The drawing under review shows one solid part. Ordinate dimensions are in mm from its lowest x, y, z. Give positions to 0.01 mm unless a question says otherwise; leave off trailing zeros. Write each loop counter-clockwise with the first axis right and the second up, starting at its lowest first coordinate (ties: lowest second). Pieces come first, ordered by that corner, then holes. Notation, with made-up numbers: (12.5, 4) -> (45.5, 4) arc R36 cw to (45.5, 38) -> close; hole circle Ø2 at (-16, -3.75). An arc over 180 degrees is marked (long way). Answer as a JSON object with one key per item and string values.
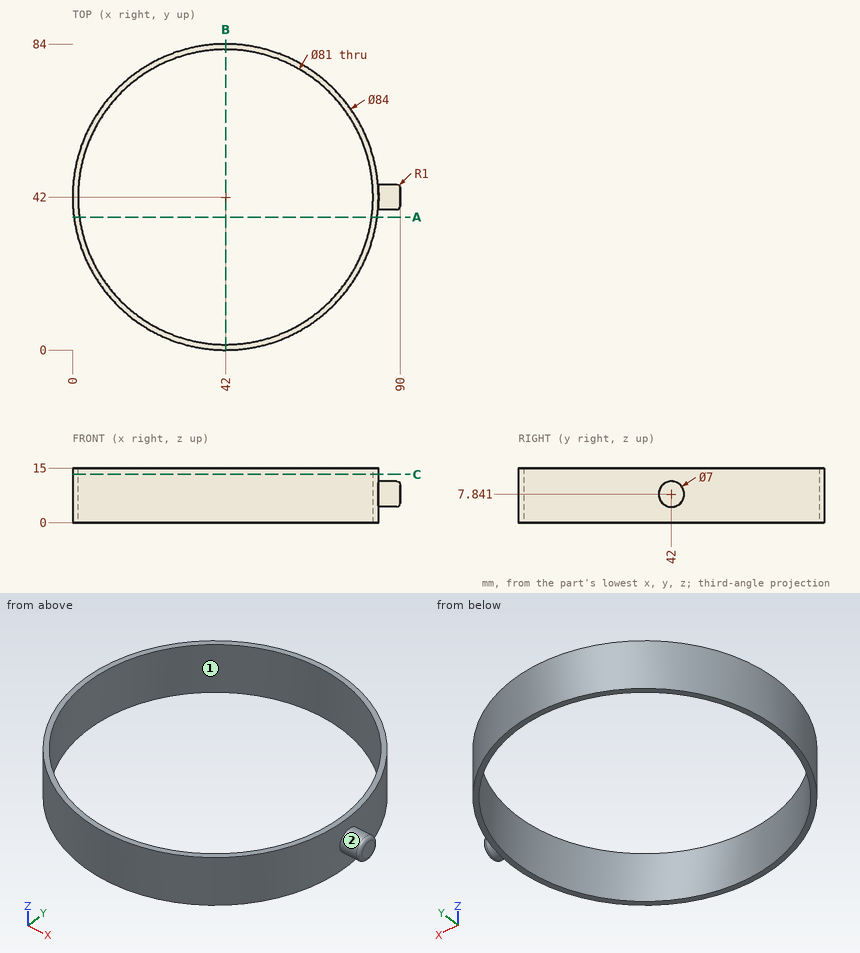
(1) We need section B-B, the plane x = 42. State the section outline as (y, z) points, then the cut area to 3 significant figures.
Here are the results:
{"outline": "(0, 0) -> (1.5, 0) -> (1.5, 15) -> (0, 15) -> close; (82.5, 0) -> (84, 0) -> (84, 15) -> (82.5, 15) -> close", "area": "45.0 mm²"}
(2) For line 1 along Y through (x, z) = (42, 7); line 2 along Y through (x, z) = (54, 7.75); line 3 along X through (y, z) = (52, 10.5) (1 decimal), list the stretches that pass through material, from the lowest coordinate up.
Here are the results:
{"line 1": "y = 0 to 1.5, 82.5 to 84", "line 2": "y = 1.75 to 3.32, 80.68 to 82.25", "line 3": "x = 1.2 to 2.8, 81.2 to 82.8"}
(3) The part is to be moulded in two halves that separate along Y. For the marked faces 1 and 2, say which applies: +Y half, -Y half, draft (parallel to the pull), parting line (faces both ways), or undercut.
Here are the results:
{"face 1": "undercut", "face 2": "parting line"}
(4) We need section C-C, the plane z = 13.25. State the section outline as (x, y) points.
Here are the results:
{"outline": "circle Ø84 at (42, 42); hole circle Ø81 at (42, 42)"}
(5) We need section A-A, the plane y = 36.5. State the section outline as (x, z) points (1 decimal).
Here are the results:
{"outline": "(0.4, 0) -> (1.9, 0) -> (1.9, 15) -> (0.4, 15) -> close; (82.1, 0) -> (83.6, 0) -> (83.6, 15) -> (82.1, 15) -> close"}
(6) Clearance check with flat-ended pins moving along their axes: pin 1 (4 mm diameter, centred on y = 26.5, z = 9, fed in from +X); pin 2 (1.5 mm diameter, centred on x = 39.5, z = 10.5, fed in from +Y); pin 3 (8 mm diameter, centred on x = 23.5, z = 8, fed in from -Y). State where each tip first meets the part, or that it passes through.
Here are the results:
{"pin 1": "stops at x = 81.77", "pin 2": "stops at y = 83.96", "pin 3": "stops at y = 2.58"}
